Geometry: final body of the model. Coordinates: model frame, mm. Round coordinates to 2 decimals unless told otherwise and drop trailing zeros. Loops run counter-clockwise (first coordinate to the right, second up) from the corner with the lowest first, then second, coordinate; pieces in that order, holes last. Notation, with made-up numbers: (-35, 50.5) - (-17, 50.5) arc R15 ccw to (-17, 57.5) - close; hole circle Ø4 at (88.5, 81.25). An arc over 180 degrees is marked (long way). Use CSV: the item, a comma, the result in double quotes.
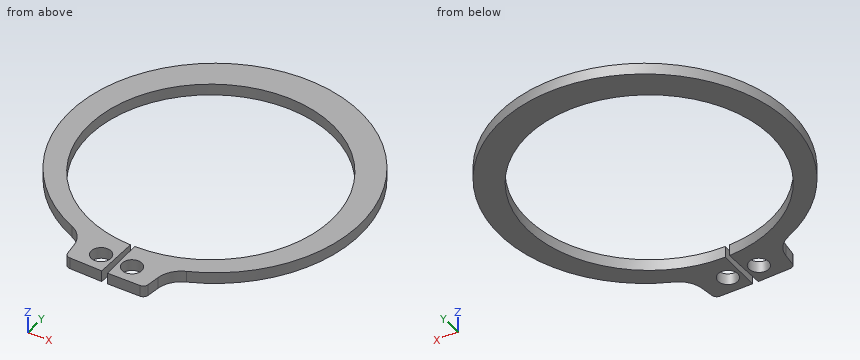
from build123d import *

# Parameters (mm, degrees)
BODYSKE_R  = 0.95
BODY_DEPTH = 1.1


with BuildPart() as part:
    # BodySke → Body (new body)
    with BuildSketch(Plane.XY):
        with BuildLine():
            Line((0.202586207, -11.748253437), (0.275, -15.947629134))
            Line((0.275, -15.947629134), (3.412936149, -15.893518744))
            ThreePointArc((3.412936149, -15.893518744), (3.737216925, -15.766656886), (3.90003789, -15.458856161))
            Line((3.90003789, -15.458856161), (4.063046444, -14.220683266))
            ThreePointArc((4.063046444, -14.220683266), (4.547351567, -13.039514962), (5.551735507, -12.251528341))
            ThreePointArc((5.551735507, -12.251528341), (0, 14.65), (-5.551735507, -12.251528341))
            ThreePointArc((-5.551735507, -12.251528341), (-4.547351567, -13.039514962), (-4.063046444, -14.220683266))
            Line((-4.063046444, -14.220683266), (-3.90003789, -15.458856161))
            ThreePointArc((-3.90003789, -15.458856161), (-3.737216925, -15.766656886), (-3.412936149, -15.893518744))
            Line((-3.412936149, -15.893518744), (-0.275, -15.947629134))
            Line((-0.275, -15.947629134), (-0.202586207, -11.748253437))
            ThreePointArc((-0.202586207, -11.748253437), (0, 11.75), (0.202586207, -11.748253437))
        make_face()
        with Locations((1.5, -14.145692807)):
            Circle(BODYSKE_R, mode=Mode.SUBTRACT)
        with Locations((-1.5, -14.145692807)):
            Circle(BODYSKE_R, mode=Mode.SUBTRACT)
    extrude(amount=-BODY_DEPTH)


solid = part.part
Item 1: Pin query (flat end, axial travel): P1, Ø1.5, axis at x = 1.5, y = -14.15, coming from the +Z side; P2, Ø2.5, axis at x = -1.5, y = -14.15, coming from the +Z side. Return the tip coordinate at first contact, or that it passes through.
Final values:
P1,"passes through"
P2,"stops at z = 0"
Item 2: Section B-B on x = -3. Return the cut outline in (y, z), plus the area to 3 significant figures.
Final values:
outline,"(-15.9, -1.1) - (-11.36, -1.1) - (-11.36, 0) - (-15.9, 0) - close; (11.36, -1.1) - (14.33, -1.1) - (14.33, 0) - (11.36, 0) - close"
area,"8.26 mm²"
Item 3: Section D-D on z = -0.65. Return the cut outline in (x, y) (3 decimals).
Final values:
outline,"(-5.552, -12.252) arc R2.5 cw to (-4.063, -14.221) - (-3.9, -15.459) arc R0.5 ccw to (-3.413, -15.894) - (-0.275, -15.948) - (-0.203, -11.748) arc R11.75 cw (long way) to (0.203, -11.748) - (0.275, -15.948) - (3.413, -15.894) arc R0.5 ccw to (3.9, -15.459) - (4.063, -14.221) arc R2.5 cw to (5.552, -12.252) arc R14.024 ccw (long way) to start; hole circle Ø1.9 at (-1.5, -14.146); hole circle Ø1.9 at (1.5, -14.146)"
Item 4: Material intervals for line 1 (Y direction, x = 2, z = -0.8); line 2 (Y direction, x = -1.5, z = -0.3); line 3 (Y direction, x = -9.5, z = -0.25), sorted ascending.
Final values:
line 1,"y = -15.92 to -14.95, -13.34 to -11.58, 11.58 to 14.51"
line 2,"y = -15.93 to -15.1, -13.2 to -11.65, 11.65 to 14.57"
line 3,"y = -9.69 to -6.91, 6.91 to 10.94"
Item 5: Section A-A on y = 0. Return the cut outline in (x, z).
Final values:
outline,"(-14.01, -1.1) - (-11.75, -1.1) - (-11.75, 0) - (-14.01, 0) - close; (11.75, -1.1) - (14.01, -1.1) - (14.01, 0) - (11.75, 0) - close"
Item 6: Section C-C on x = 1.5. Return the cut outline in (y, z).
Final values:
outline,"(-15.93, -1.1) - (-15.1, -1.1) - (-15.1, 0) - (-15.93, 0) - close; (-13.2, -1.1) - (-11.65, -1.1) - (-11.65, 0) - (-13.2, 0) - close; (11.65, -1.1) - (14.57, -1.1) - (14.57, 0) - (11.65, 0) - close"
